from build123d import *

# Parameters (mm, degrees)
SKETCH1_R           = 5.08
BASE_EXTRUDE_DEPTH  = 64.77
FILLET1_R           = 3.302
SKETCH4_W           = 2.794
SKETCH4_H           = 33.0835
BOSS_EXTRUDE1_DEPTH = 1.016
CIRPATTERN1_COUNT   = 3


with BuildPart() as part:
    # Sketch1 → Base-Extrude (new body)
    with BuildSketch(Plane(origin=(0, 0, 0), x_dir=(1, 0, 0), z_dir=(0, 1, 0))):
        with Locations(Location((0, 0, 0), (0, 0, 270))):
            Circle(SKETCH1_R)
    extrude(amount=BASE_EXTRUDE_DEPTH)

    # Fillet1
    fillet1_edges = [part.edges().sort_by_distance(p)[0] for p in [
        (0, 64.77, -5.08),
    ]]
    fillet(fillet1_edges, radius=FILLET1_R)

    # Sketch4 → Cut-Revolve1 (revolve, cut)
    with BuildSketch(Plane.XY, mode=Mode.PRIVATE) as cut_revolve1_sk:
        with Locations((-1.397, 16.54175)):
            Rectangle(SKETCH4_W, SKETCH4_H)
    revolve(cut_revolve1_sk.sketch.rotate(Axis((0, 33.0835, 0), (0, 1, 0)), 180), axis=Axis((0, 33.0835, 0), (0, 1, 0)), mode=Mode.SUBTRACT)

    # Sketch3 → Boss-Extrude1 (add, symmetric)
    with BuildSketch(Plane.XY):
        with BuildLine():
            Line((-4.826, 0.254), (-12.7, 0.254))
            ThreePointArc((-12.7, 0.254), (-15.465187802, 1.868755974), (-15.417711968, 5.070543987))
            Line((-15.417711968, 5.070543987), (-4.826, 22.606))
            Line((-4.826, 22.606), (-4.826, 0.254))
        make_face()
    boss_extrude1 = extrude(amount=BOSS_EXTRUDE1_DEPTH, both=True)

    # CirPattern1: Boss-Extrude1 ×3 about axis
    cirpattern1_axis = Axis((0, 0, 0), (0, 1, 0))
    for i in range(1, CIRPATTERN1_COUNT):
        add(boss_extrude1.rotate(cirpattern1_axis, i * 360 / CIRPATTERN1_COUNT))


solid = part.part
Check sheet for the modelled part. Datum: model origin and axes. Units: mm. A direction names the side the tool comes from. Give positions to 0.01 mm unless a question says otherwise; leave off trailing zeros. Loops run counter-clockwise (first coordinate to the right, second up) from the corner with the lowest first, then second, coordinate; pieces in that order, holes last. Notation, with made-up numbers: M 35.5,-31 L 80.5,-31 A25 cw 80.5,7 Z; hole C 74.5,22 d10. An arc over 180 degrees is marked long. Answer as a JSON object with one key per item and string values. Group by question number.
Q1. Material ranges on line 1 along Y through (x, z) = (-1, 1); line 2 along Z through (x, y) = (-1, 29); line 3 along X through (y, z) = (7.5, -6), recorded low to high. Write a range as [from, to].
Q2. Cross-section at C-C on y = 46. Record the cut outline in (x, z), then the cut area to 3 significant figures.
Q3. Go/stop test with flat-tipped pins: P1, Ø1.7, axis at x = 5, z = -6, coming from the -Y side; P2, Ø5, axis at x = 5.5, y = 31, coming from the -Z side; P3, Ø1, axis at x = -1.5, y = 17.5, coming from the +Z side. Record where each tip stops, or that it passes through.
Q4. Cross-section at A-A on y = 11. Record the cut outline in (x, z), then the cut area to 3 significant figures.
Q5. Access from +Z, -Z, +X, -X, +Y, -Y to the whole of each face (thin tool, end or side, straight path). Record for faces 5 (the flat face through (0, 33.084, 0)), 6 (the flat face through (-9, 9, 1.016)), 7 (the flat face through (4, 0.254, -8)).
Q6. Release check for a two-part mould opening along Z. For faces 1 (the flat face through (5.15, 13.59, 8.89)), 2 (the flat face through (4, 0.254, 8)), 3 (the flat face through (5.45, 9, -7.41)), 4 (the flat face through (5.45, 9, 7.41)) record: released by +Z, released by -Z, zero draft, split by the parting line, or undercut.
Q7. Cross-section at D-D on x = -5.75. Record the cut outline in (y, z).
Q8. Cross-section at B-B on z = -9.5. Record the cut outline in (x, y), then the cut area to 3 significant figures.
Evaluation:
{
 "1": {"line 1": "y = [33.08, 64.77]", "line 2": "z = [-4.98, -2.61], [2.61, 4.98]", "line 3": "x = [2.29, 4.64]"},
 "2": {"outline": "C 0,0 d10.16", "area": "81.1 mm2"},
 "3": {"P1": "stops at y = 0.25", "P2": "stops at z = -4.1", "P3": "stops at z = 4.98"},
 "4": {"outline": "M -11.84,-1.02 L -4.98,-1.02 A5.08 ccw 1.61,-4.82 L 5.04,-10.76 L 6.8,-9.74 L 3.37,-3.8 A5.08 ccw 3.37,3.8 L 6.8,9.74 L 5.04,10.76 L 1.61,4.82 A5.08 ccw -4.98,1.02 L -11.84,1.02 Z; hole C 0,0 d5.59", "area": "97.9 mm2"},
 "5": {"face 5": "-Y", "face 6": "+Z, -X, +Y, -Y", "face 7": "-Z, +X, -Y"},
 "6": {"face 1": "released by +Z", "face 2": "zero draft", "face 3": "undercut", "face 4": "undercut"},
 "7": {"outline": "M 0.25,-1.02 L 21.08,-1.02 L 21.08,1.02 L 0.25,1.02 Z"},
 "8": {"outline": "M 4.31,0.25 L 6.66,0.25 L 6.66,11.46 L 4.31,13.41 Z", "area": "28.6 mm2"}
}
